```python
from build123d import *

# Parameters (mm, degrees)
F0_R     = 14.413893
F1_DEPTH = 25
F3_DEPTH = 5


with BuildPart() as f1:
    # F0 (on Top) → F1 (new body)
    with BuildSketch(Plane.XY):
        Circle(F0_R)
        Polygon((6.449648, 6.660601), (8.993074, -2.255258), (2.543426, -8.915859), (-6.449648, -6.660601), (-8.993074, 2.255258), (-2.543426, 8.915859), align=None, mode=Mode.SUBTRACT)
    extrude(amount=F1_DEPTH)

    # F2 (on face) → F3 (join)
    with BuildSketch(Plane.XY.offset(25)):
        with BuildLine():
            Line((-14.413893, 63.413893), (-14.413893, 0))
            ThreePointArc((-14.413893, 0), (0, 14.413893), (14.413893, 0))
            Line((14.413893, 0), (14.413893, 63.413893))
            Line((14.413893, 63.413893), (4, 63.413893))
            ThreePointArc((4, 63.413893), (0, 59.413893), (-4, 63.413893))
            Line((-4, 63.413893), (-14.413893, 63.413893))
        make_face()
        with BuildLine():
            ThreePointArc((14.413893, 0), (0, 14.413893), (-14.413893, 0))
            ThreePointArc((-14.413893, 0), (0, -14.413893), (14.413893, 0))
        make_face()
        Polygon((-2.543426, 8.915859), (6.449648, 6.660601), (8.993074, -2.255258), (2.543426, -8.915859), (-6.449648, -6.660601), (-8.993074, 2.255258), align=None, mode=Mode.SUBTRACT)
        with BuildLine():
            ThreePointArc((14.413893, 63.413893), (0, 77.827787), (-14.413893, 63.413893))
            Line((-14.413893, 63.413893), (-4, 63.413893))
            ThreePointArc((-4, 63.413893), (0, 67.413893), (4, 63.413893))
            Line((4, 63.413893), (14.413893, 63.413893))
        make_face()
    extrude(amount=F3_DEPTH)


solid = f1.part
```
CAD build for the part. Positions are in the model's coordinates, mm. Give positions to 0.01 mm unless a question says otherwise; leave off trailing zeros. Order: outer loops, then holes, each group sorted by start corner. A loop starts at its lowest first (then second) coordinate and runs counter-clockwise, first axis right, second up. Notation, with made-up numbers: M 30,86 L 70,86 A12 cw 70,100 Z; hole C -37.75,-16.75 d9. An arc over 180 degrees is marked long. Put each result on its own line as item: value. Start each with the question number.
(1) Flat gauge pins, fed straight in: pin 1 Ø10 at (y, z) = (6, 6.5) entering from +X; pin 2 Ø7 at (x, y) = (0, 63.41) entering from -Z; pin 3 Ø14.5 at (x, y) = (-4, 22.5) entering from -Z. Where does each tip first touch, or does it go through?
(2) Saw through at B-B, the plane x = 0. Write the cut outline in (y, z).
(3) Drill centre lines: line 1 along Y through (x, z) = (0, 26.5); line 2 along Z through (x, y) = (8.5, 57); line 3 along Y through (x, z) = (-6.25, 7.25). Where is each one in solid material? Low to high.
(4) Saw through at C-C, the plane z = 22. Write the cut outline in (x, y), then the cut area to 3 significant figures.
(5) Saw through at A-A, the plane z = 27.5. Write the cut outline in (x, y), then the cut area to 3 significant figures.
(6) Saw through at D-D, the plane y = 64.5. Write the cut outline in (x, z), then the cut area to 3 significant figures.
Check result:
1. pin 1: stops at x = 14.38
1. pin 2: passes through
1. pin 3: stops at z = 25
2. outline: M -14.41,0 L -8.28,0 L -8.28,30 L -14.41,30 Z; M 8.28,0 L 14.41,0 L 14.41,25 L 59.41,25 L 59.41,30 L 8.28,30 Z; M 67.41,25 L 77.83,25 L 77.83,30 L 67.41,30 Z
3. line 1: y = -14.41 to -8.28, 8.28 to 59.41, 67.41 to 77.83
3. line 2: z = 25 to 30
3. line 3: y = -12.99 to -6.71, 5.09 to 12.99
4. outline: C 0,0 d28.83; hole M -8.99,2.26 L -6.45,-6.66 L 2.54,-8.92 L 8.99,-2.26 L 6.45,6.66 L -2.54,8.92 Z
4. area: 429 mm2
5. outline: M -14.41,0 A14.41 ccw 14.41,0 L 14.41,63.41 A14.41 ccw -14.41,63.41 Z; hole M -8.99,2.26 L -6.45,-6.66 L 2.54,-8.92 L 8.99,-2.26 L 6.45,6.66 L -2.54,8.92 Z; hole C 0,63.41 d8
5. area: 2,210 mm2
6. outline: M -14.37,25 L -3.85,25 L -3.85,30 L -14.37,30 Z; M 3.85,25 L 14.37,25 L 14.37,30 L 3.85,30 Z
6. area: 105 mm2
